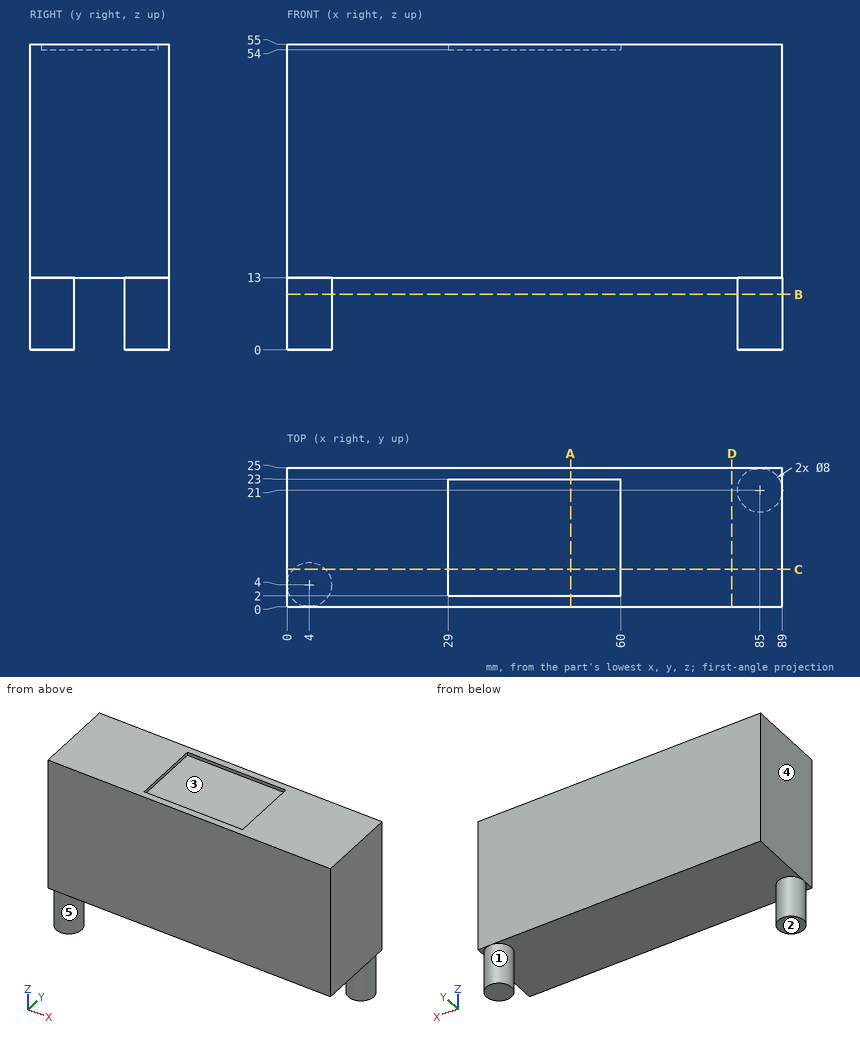
The drawing under review shows one solid part. Ordinate dimensions are in mm from its lowest x, y, z. A direction names the side the tool comes from. Coordinates: 2 decimals unless noted, no trailing zeros. Order: outer loops, then holes, each group sorted by start corner. A loop starts at its lowest first (then second) coordinate and runs counter-clockwise, first axis right, second up. Notation, with made-up numbers: M 16,-32 L 61,-32 A16 ccw 61,-20 Z; hole C -17.75,-38.75 d6. An arc over 180 degrees is marked long. One line per question, with ' | ' between items.
(1) The part is to be moulded in two halves that separate along X. For the marked faces 3, 4 and 5, say which applies: +X half, -X half, draft (parallel to the pull), parting line (faces both ways), or undercut.
Geometry results:
face 3: undercut | face 4: -X half | face 5: parting line
(2) Add section A-A, the plane x = 51. Write out the cut boundary in (y, z), then the cut area to 3 significant figures.
Geometry results:
outline: M 0,13 L 25,13 L 25,55 L 23,55 L 23,54 L 2,54 L 2,55 L 0,55 Z | area: 1,030 mm²
(3) Add section D-D, the plane x = 80. Write out the cut boundary in (y, z), then the cut area to 3 significant figures.
Geometry results:
outline: M 0,13 L 25,13 L 25,55 L 0,55 Z | area: 1,050 mm²
(4) Insertion check: pin 1 (8 mm diameter, centred on x = 68, y = 20.5, fed in from -Z); pin 2 (4.5 mm diameter, centred on x = 1, y = 1, fed in from -Z). Each pin has a flat end and moves straight along its axis. Give the tip position at first contact, or say it passes through.
Geometry results:
pin 1: stops at z = 13 | pin 2: stops at z = 0
(5) Machinability: for the marked faces 1 and 2, which of the approach directions +Z, -Z, +X, -X, +Y, -Y give a long, thin tool a straight path to every point of the face, cutting with its end or side? Answer none if there is none.
Geometry results:
face 1: -Z | face 2: -Z, +X, -X, +Y, -Y
(6) Add section B-B, the plane z = 10. Write out the cut boundary in (x, y).
Geometry results:
outline: C 4,4 d8; C 85,21 d8
(7) For probe 1 along Z at (x, y) = (65.5, 10.75); probe 2 along Z at (x, y) = (38.5, 17.75); probe 3 along X at (y, z) = (23.25, 10), list the stretches that pass through material, from the lowest coordinate up. Write a range as from..to.
Geometry results:
probe 1: z = 13..55 | probe 2: z = 13..54 | probe 3: x = 81.69..88.31
(8) Add section C-C, the plane y = 6.75. Write out the cut boundary in (x, z), then the cut area to 3 significant figures.
Geometry results:
outline: M 0,13 L 1.1,13 L 1.1,0 L 6.9,0 L 6.9,13 L 89,13 L 89,55 L 60,55 L 60,54 L 29,54 L 29,55 L 0,55 Z | area: 3,780 mm²
